Geometry: final body of the model. Coordinates: model frame, mm. Face numbers are marked on the shaded views. A direction names the side the tool comes from. Round coordinates to 2 decimals unless told otherwise and drop trailing zeros. Order: outer loops, then holes, each group sorted by start corner. A loop starts at its lowest first (then second) coordinate and runs counter-clockwise, first axis right, second up. Notation, with made-up numbers: (55.5, 18) - (79.5, 18) arc R25 ccw to (79.5, 33) - close; hole circle Ø11 at (86, 64). An arc over 180 degrees is marked (long way). Put each result on its own line as item: value. Start each with the question number.
(1) Section D-D (y = 30.25). Count the separate pieces of the cut face and the enclosed holes in it, and give its area (3 significant figures).
(2) Material intervals for L1, parallel to Z at x = 10, y = 33.7; L2, parallel to Z at x = -10, y = 28.5; L3, parallel to X at y = 33, z = 20, sorted ascending. Write a range as [from, to].
(3) Section A-A (z = 41.5). Output: boundary loops of the cut face in (x, y), and give its area (3 significant figures).
(4) Section B-B (y = 24.5). Output: boundary loops of the cut face in (x, z), and give its area (3 significant figures).
(5) Section C-C (x = -19). Output: boundary loops of the cut face in (y, z).
(6) Pin query (flat end, axial travel): P1, Ø0.9, axis at x = 2, y = 25, coming from the -Z side; P2, Ø5.5, axis at y = 30, z = 18, coming from the +X side; P3, Ø8.5, axis at x = 10, z = 35.5, coming from the +Y side. Return the tip coordinate at first contact, or that it passes through.
(7) Pull-direction query (Z, two-part tool) for the marked faces 4, 5 and 6; classes: released by +Z, released by -Z, zero draft, split by the parting line, or undercut.
(8) Access query for the marked faces 1, 2 and 3. Directions: +Z, -Z, +X, -X, +Y, -Y. A direction counts if a zero-diameter tool reaches every point of the face in a straight line with its end or side. Return the directions, or none.
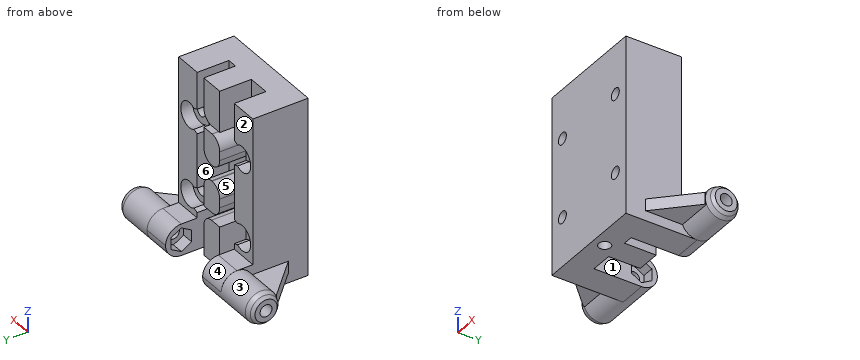
from build123d import *

# Parameters (mm, degrees)
SKETCH008_W     = 28
SKETCH008_H     = 45
SKETCH008_R     = 1.5
PAD003_DEPTH    = 6
SKETCH009_W     = 7
SKETCH009_H     = 45
SKETCH009_R     = 1.5
SKETCH009_W_2   = 6
SKETCH009_H_2   = 10.5
SKETCH009_H_3   = 8
PAD004_DEPTH    = 8
FILLET002_R     = 2.9
SKETCH011_W     = 7
SKETCH011_H     = 8
PAD005_DEPTH    = 8
FILLET003_R     = 3.99
SKETCH012_R     = 3.99
PAD006_DEPTH    = 11
SKETCH013_R     = 3.99
PAD007_DEPTH    = 11
SKETCH014_R     = 1.5
POCKET001_DEPTH = 52
CHAMFER001_SIZE = 1.2
SKETCH015_W     = 3
SKETCH015_H     = 10
PAD008_DEPTH    = 9
SKETCH016_W     = 3
SKETCH016_H     = 10
PAD009_DEPTH    = 9
CHAMFER002_SIZE = 8.9999
CHAMFER003_SIZE = 0.7
POCKET002_DEPTH = 3
POCKET003_DEPTH = 3
SKETCH019_R     = 1.5
POCKET004_DEPTH = 15
SKETCH020_R     = 3.2
POCKET005_DEPTH = 3
CHAMFER004_SIZE = 2


with BuildPart() as part:
    # Sketch008 → Pad003 (new body)
    with BuildSketch(Plane.XZ):
        with Locations((14, 22.5)):
            Rectangle(SKETCH008_W, SKETCH008_H)
        with Locations((4, 32.5)):
            Circle(SKETCH008_R, mode=Mode.SUBTRACT)
        with Locations((24, 32.5)):
            Circle(SKETCH008_R, mode=Mode.SUBTRACT)
        with Locations((4, 12.5)):
            Circle(SKETCH008_R, mode=Mode.SUBTRACT)
        with Locations((24, 12.5)):
            Circle(SKETCH008_R, mode=Mode.SUBTRACT)
    extrude(amount=PAD003_DEPTH)

    # Sketch009 (on Face9 of Pad003) → Pad004 (join)
    with BuildSketch(Plane(origin=(0, 0, 0), x_dir=(1, 0, 0), z_dir=(0, 1, 0))):
        with Locations((3.5, -22.5)):
            Rectangle(SKETCH009_W, SKETCH009_H)
        with Locations((4, -12.5)):
            Circle(SKETCH009_R, mode=Mode.SUBTRACT)
        with Locations((4, -32.5)):
            Circle(SKETCH009_R, mode=Mode.SUBTRACT)
        with Locations((24.5, -22.5)):
            Rectangle(SKETCH009_W, SKETCH009_H)
        with Locations((24, -12.5)):
            Circle(SKETCH009_R, mode=Mode.SUBTRACT)
        with Locations((24, -32.5)):
            Circle(SKETCH009_R, mode=Mode.SUBTRACT)
        with Locations((15.5, -5.25)):
            Rectangle(SKETCH009_W_2, SKETCH009_H_2)
        with Locations((15.5, -16.5)):
            Rectangle(SKETCH009_W_2, SKETCH009_H_3)
        with Locations((15.5, -28.5)):
            Rectangle(SKETCH009_W_2, SKETCH009_H_3)
        with Locations((15.5, -39.75)):
            Rectangle(SKETCH009_W_2, SKETCH009_H_2)
    extrude(amount=PAD004_DEPTH)

    # Fillet002
    fillet002_edges = [part.edges().sort_by_distance(p)[0] for p in [
        (12.5, 4, 24.5),
        (18.5, 4, 24.5),
        (12.5, 4, 32.5),
        (18.5, 4, 34.5),
        (18.5, 4, 20.5),
        (12.5, 4, 20.5),
        (12.5, 4, 12.5),
        (18.5, 4, 10.5),
    ]]
    fillet(fillet002_edges, radius=FILLET002_R)

    # Sketch011 (on Face36 of Fillet002) → Pad005 (join)
    with BuildSketch(Plane(origin=(0, 8, 0), x_dir=(1, 0, 0), z_dir=(0, 1, 0))):
        with Locations((3.5, -4)):
            Rectangle(SKETCH011_W, SKETCH011_H)
        with Locations((24.5, -4)):
            Rectangle(SKETCH011_W, SKETCH011_H)
    extrude(amount=PAD005_DEPTH)

    # Fillet003
    fillet003_edges = [part.edges().sort_by_distance(p)[0] for p in [
        (3.5, 16, 8),
        (3.5, 16, 0),
        (24.5, 16, 0),
        (24.5, 16, 8),
    ]]
    fillet(fillet003_edges, radius=FILLET003_R)

    # Sketch012 (on Face8 of Fillet003) → Pad006 (join)
    with BuildSketch(Plane(origin=(0, 0, 0), x_dir=(0, 0, -1), z_dir=(-1, 0, 0))):
        with Locations((-3.99, -12.01)):
            Circle(SKETCH012_R)
    extrude(amount=PAD006_DEPTH)

    # Sketch013 (on Face68 of Pad006) → Pad007 (join)
    with BuildSketch(Plane(origin=(28, 0, 0), x_dir=(0, 0, 1), z_dir=(1, 0, 0))):
        with Locations((3.99, -12.01)):
            Circle(SKETCH013_R)
    extrude(amount=PAD007_DEPTH)

    # Sketch014 (on Face70 of Pad007) → Pocket001 (cut)
    with BuildSketch(Plane(origin=(39, 0, 0), x_dir=(0, 0, 1), z_dir=(1, 0, 0))):
        with Locations((3.99, -12.01)):
            Circle(SKETCH014_R)
    extrude(amount=-POCKET001_DEPTH, mode=Mode.SUBTRACT)

    # Chamfer001
    chamfer001_edges = [part.edges().sort_by_distance(p)[0] for p in [
        (-11, 12.01, 7.98),
        (39, 12.01, 0),
    ]]
    chamfer(chamfer001_edges, length=CHAMFER001_SIZE)

    # Sketch015 (on Face10 of Chamfer001) → Pad008 (join)
    with BuildSketch(Plane(origin=(0, 0, 0), x_dir=(0, 0, -1), z_dir=(-1, 0, 0))):
        with Locations((-4, -4)):
            Rectangle(SKETCH015_W, SKETCH015_H)
    extrude(amount=PAD008_DEPTH)

    # Sketch016 (on Face62 of Pad008) → Pad009 (join)
    with BuildSketch(Plane(origin=(28, 0, 0), x_dir=(0, 0, 1), z_dir=(1, 0, 0))):
        with Locations((4, -4)):
            Rectangle(SKETCH016_W, SKETCH016_H)
    extrude(amount=PAD009_DEPTH)

    # Chamfer002
    chamfer002_edges = [part.edges().sort_by_distance(p)[0] for p in [
        (37, -1, 4),
        (-9, -1, 4),
    ]]
    chamfer(chamfer002_edges, length=CHAMFER002_SIZE)

    # Chamfer003
    chamfer003_edges = [part.edges().sort_by_distance(p)[0] for p in [
        (-9.8, 12.01, 7.98),
        (37.8, 12.01, 0),
    ]]
    chamfer(chamfer003_edges, length=CHAMFER003_SIZE)

    # Sketch017 (on Face75 of Chamfer003) → Pocket002 (cut)
    with BuildSketch(Plane(origin=(21, 0, 0), x_dir=(0, 0, -1), z_dir=(-1, 0, 0))):
        Polygon((-2.49, -14.608076), (-0.99, -12.01), (-2.49, -9.411924), (-5.49, -9.411924), (-6.99, -12.01), (-5.49, -14.608076), align=None)
    extrude(amount=-POCKET002_DEPTH, mode=Mode.SUBTRACT)

    # Sketch018 (on Face16 of Pocket002) → Pocket003 (cut)
    with BuildSketch(Plane(origin=(7, 0, 0), x_dir=(0, 0, 1), z_dir=(1, 0, 0))):
        Polygon((5.49, -14.608076), (6.99, -12.01), (5.49, -9.411924), (2.49, -9.411924), (0.99, -12.01), (2.49, -14.608076), align=None)
    extrude(amount=-POCKET003_DEPTH, mode=Mode.SUBTRACT)

    # Sketch019 (on Face22 of Pocket003) → Pocket004 (cut)
    with BuildSketch(Plane(origin=(0, 0, 0), x_dir=(1, 0, 0), z_dir=(0, 0, -1))):
        with Locations((15.5, 3)):
            Circle(SKETCH019_R)
    extrude(amount=-POCKET004_DEPTH, mode=Mode.SUBTRACT)

    # Sketch020 (on Face32 of Pocket004) → Pocket005 (cut)
    with BuildSketch(Plane(origin=(0, 8, 0), x_dir=(1, 0, 0), z_dir=(0, 1, 0))):
        with Locations((4, -12.5)):
            Circle(SKETCH020_R)
        with Locations((4, -32.5)):
            Circle(SKETCH020_R)
        with Locations((24, -32.5)):
            Circle(SKETCH020_R)
        with Locations((24, -12.5)):
            Circle(SKETCH020_R)
    extrude(amount=-POCKET005_DEPTH, mode=Mode.SUBTRACT)

    # Chamfer004
    chamfer004_edges = [part.edges().sort_by_distance(p)[0] for p in [
        (7, 6.5, 11.386447),
        (7, 6.5, 13.613553),
        (21, 6.5, 11.386447),
        (7, 6.5, 31.386447),
        (21, 6.5, 31.386447),
        (7, 6.5, 33.613553),
        (21, 6.5, 33.613553),
        (21, 6.5, 13.613553),
    ]]
    chamfer(chamfer004_edges, length=CHAMFER004_SIZE)


with BuildPart() as part_1:
    # Body006 placement: moved
    add(part.part.moved(Location((-14, 27.5, 3))))


solid = part_1.part
Checks:
1. separate pieces: 6
1. enclosed holes: 4
1. area: 832 mm²
2. L1: z = [3, 12.3], [18.7, 32.3], [38.7, 48]
2. L2: z = [3, 14], [17, 34], [37, 48]
2. L3: x = [-14, -7], [-1.5, 4.5], [7, 14]
3. outline: (-14, 21.5) - (14, 21.5) - (14, 35.5) - (7, 35.5) - (7, 27.5) - (4.5, 27.5) - (4.5, 35.5) - (-1.5, 35.5) - (-1.5, 27.5) - (-7, 27.5) - (-7, 35.5) - (-14, 35.5) - close
3. area: 328 mm²
4. outline: (-14, 3) - (0, 3) - (0, 18) - (3, 18) - (3, 3) - (14, 3) - (14, 48) - (-14, 48) - close; hole circle Ø3 at (-10, 15.5); hole circle Ø3 at (-10, 35.5); hole circle Ø3 at (10, 15.5); hole circle Ø3 at (10, 35.5)
4. area: 1,190 mm²
5. outline: (31.5, 5.5) - (35.81, 5.5) arc R3.99 ccw (long way) to (35.82, 8.5) - (31.5, 8.5) - close; hole circle Ø3 at (39.51, 6.99)
6. P1: stops at z = 18
6. P2: stops at x = 14
6. P3: stops at y = 35.5
7. face 4: released by +Z
7. face 5: undercut
7. face 6: zero draft
8. face 1: +Z, -Z, +Y
8. face 2: +Z, +X, -X, +Y
8. face 3: -X
